CAD build for the part. Positions are in the model's coordinates, mm. Give positions to 0.01 mm unless a question says otherwise; leave off trailing zeros. Loops run counter-clockwise (first coordinate to the right, second up) from the corner with the lowest first, then second, coordinate; pieces in that order, holes last. Notation, with made-up numbers: (-38.75, 16) - (13.25, 16) arc R13 cw to (13.25, 36) - close; hole circle Ø5 at (58.5, 0). An arc over 180 degrees is marked (long way). Return JSON: item names as keys, results as strings.
Autodesk Inventor part; units mm, degrees
ref_plane "YZ Plane" through (0, 0, 0) normal (1, 0, 0) x (0, 1, 0)
ref_plane "XZ Plane" through (0, 0, 0) normal (0, 1, 0) x (-1, 0, 0)
ref_plane "XY Plane" through (0, 0, 0) normal (0, 0, 1) x (1, 0, 0)
ref_plane "Work Plane1" through (-190.5, 0, 0) normal (0, 0, 1) x (1, 0, 0)
sketch "Sketch1" plane through (-190.5, 0, 0) normal (0, 0, 1) x (1, 0, 0)
  circle A0 centre (0, 0) radius 2.4638
  circle A1 centre (76.2, 0) radius 2.4638
  circle A2 centre (114.3, 0) radius 2.4638
  circle A3 centre (190.5, 0) radius 2.4638
  circle A4 centre (0, 0) radius 6.35
  circle A5 centre (190.5, 0) radius 6.35
  line L0 (0, 6.35) -> (190.5, 6.35)
  line L1 (190.5, -6.35) -> (0, -6.35)
  point P0 (190.5, 0)
  dimension "d0" = 12.7
  dimension "d1" = 12.7
extrude "Extrusion1" add sketch "Sketch1" along normal blind 1.5875
properties part number "bottomSled"
1. Cut at C-C, the plane x = -114.3. Write the cut outline in (y, z), plus the area to 3 significant figures.
Values follow:
{"outline": "(-6.35, 0) - (-2.46, 0) - (-2.46, 1.59) - (-6.35, 1.59) - close; (2.46, 0) - (6.35, 0) - (6.35, 1.59) - (2.46, 1.59) - close", "area": "12.3 mm²"}
2. Cut at A-A, the plane y = 0. Write the cut outline in (x, z).
Values follow:
{"outline": "(-196.85, 0) - (-192.96, 0) - (-192.96, 1.59) - (-196.85, 1.59) - close; (-188.04, 0) - (-116.76, 0) - (-116.76, 1.59) - (-188.04, 1.59) - close; (-111.84, 0) - (-78.66, 0) - (-78.66, 1.59) - (-111.84, 1.59) - close; (-73.74, 0) - (-2.46, 0) - (-2.46, 1.59) - (-73.74, 1.59) - close; (2.46, 0) - (6.35, 0) - (6.35, 1.59) - (2.46, 1.59) - close"}
3. Drill centre lines: probe 1 along Y at (x, z) = (-76.2, 1); probe 2 along X at (y, z) = (1.5, 1.3). Where is each one in solid material? Low to high.
Values follow:
{"probe 1": "y = -6.35 to -2.46, 2.46 to 6.35", "probe 2": "x = -196.67 to -192.45, -188.55 to -116.25, -112.35 to -78.15, -74.25 to -1.95, 1.95 to 6.17"}
4. Drop a flat-ended pin along its axis: P1, Ø6.5, axis at x = -114.3, y = 0, coming from the +Z side. Give the stop position or say it passes through.
Values follow:
{"P1": "stops at z = 1.59"}
5. Cut at B-B, the plane z = 0.6. Write the cut outline in (x, y), plus the area to 3 significant figures.
Values follow:
{"outline": "(-190.5, -6.35) - (0, -6.35) arc R6.35 ccw to (0, 6.35) - (-190.5, 6.35) arc R6.35 ccw to start; hole circle Ø4.93 at (-190.5, 0); hole circle Ø4.93 at (-114.3, 0); hole circle Ø4.93 at (-76.2, 0); hole circle Ø4.93 at (0, 0)", "area": "2,470 mm²"}
6. Pull direction Y, two halves, no side cores. Call faces 1 (the face through (6.35, 0.14, 0.78)), 2 (the face through (-192.96, -0.11, 0.78)), 3 (the face through (-97, 0, 0)): +Y half, -Y half, draft (parallel to the pull), parting line (faces both ways), or undercut.
Values follow:
{"face 1": "parting line", "face 2": "undercut", "face 3": "draft"}
